Could you check a few things on this model? Use its own coordinates, in mm. A direction names the side the tool comes from. Give positions to 0.01 mm unless a question says otherwise; leave off trailing zeros. Order: outer loops, then holes, each group sorted by start corner. A loop starts at its lowest first (then second) coordinate and runs counter-clockwise, first axis right, second up.
from build123d import *

# Parameters (mm, degrees)
ESQUISSE1_R             = 1.55
BOSS_EXTRU_1_DEPTH      = 8
ENL_V_MAT_EXTRU_1_DEPTH = 4
ESQUISSE3_R             = 4
ENL_V_MAT_EXTRU_2_DEPTH = 38


with BuildPart() as part:
    # Esquisse1 → Boss.-Extru.1 (new body)
    with BuildSketch(Plane.XY):
        with BuildLine():
            Line((-2.034299831, 64.480985332), (56.965700169, 64.480985332))
            Line((56.965700169, 64.480985332), (56.965700169, 46.626034607))
            ThreePointArc((56.965700169, 46.626034607), (56.941837013, 44.504848488), (59.063023131, 44.480985332))
            Line((59.063023131, 44.480985332), (62.935403121, 44.480985332))
            ThreePointArc((62.935403121, 44.480985332), (65.056723464, 44.480985332), (65.056723464, 46.602305676))
            Line((65.056723464, 46.602305676), (65.056723464, 64.480985332))
            Line((65.056723464, 64.480985332), (249.965700169, 64.480985332))
            Line((249.965700169, 64.480985332), (249.965700169, 34.480985332))
            Line((249.965700169, 34.480985332), (244.087020512, 34.480985332))
            ThreePointArc((244.087020512, 34.480985332), (241.965700169, 34.480985332), (241.965700169, 32.359664989))
            Line((241.965700169, 32.359664989), (241.965700169, -3.397694324))
            ThreePointArc((241.965700169, -3.397694324), (241.965700169, -5.519014668), (244.087020512, -5.519014668))
            Line((244.087020512, -5.519014668), (249.965700169, -5.519014668))
            Line((249.965700169, -5.519014668), (249.965700169, -35.519014668))
            Line((249.965700169, -35.519014668), (47.965700169, -35.519014668))
            Line((47.965700169, -35.519014668), (47.965700169, 12.359664989))
            ThreePointArc((47.965700169, 12.359664989), (47.965700169, 14.480985332), (45.844379825, 14.480985332))
            Line((45.844379825, 14.480985332), (42.087020512, 14.480985332))
            ThreePointArc((42.087020512, 14.480985332), (39.965700169, 14.480985332), (39.965700169, 12.359664989))
            Line((39.965700169, 12.359664989), (39.965700169, -35.519014668))
            Line((39.965700169, -35.519014668), (-50.034299831, -35.519014668))
            Line((-50.034299831, -35.519014668), (-50.034299831, 22.512874652))
            Line((-50.034299831, 22.512874652), (-2.034299831, 64.480985332))
        make_face()
        with Locations((245.965700169, 49.480985332)):
            Circle(ESQUISSE1_R, mode=Mode.SUBTRACT)
        with Locations((245.965700169, -20.519014668)):
            Circle(ESQUISSE1_R, mode=Mode.SUBTRACT)
        with Locations((43.965700169, 39.480985332)):
            Circle(ESQUISSE1_R, mode=Mode.SUBTRACT)
    extrude(amount=BOSS_EXTRU_1_DEPTH)

    # Esquisse2 → Enlèv. mat.-Extru.1 (cut)
    with BuildSketch(Plane(origin=(0, 0, 0), x_dir=(-1, 0, 0), z_dir=(0, 0, -1))):
        with BuildLine():
            Line((-245.965700169, 64.480985332), (-60.965700169, 64.480985332))
            Line((-60.965700169, 64.480985332), (-60.965700169, 52.480985332))
            Line((-60.965700169, 52.480985332), (-243.844379825, 52.480985332))
            ThreePointArc((-243.844379825, 52.480985332), (-245.965700169, 52.480985332), (-245.965700169, 54.602305676))
            Line((-245.965700169, 54.602305676), (-245.965700169, 64.480985332))
        make_face()
    extrude(amount=-ENL_V_MAT_EXTRU_1_DEPTH, mode=Mode.SUBTRACT)

    # Esquisse3 → Enlèv. mat.-Extru.2 (cut)
    with BuildSketch(Plane(origin=(0, 0, 0), x_dir=(-1, 0, 0), z_dir=(0, 0, -1))):
        with Locations((30.034299831, -15.519014668)):
            Circle(ESQUISSE3_R)
    extrude(amount=-ENL_V_MAT_EXTRU_2_DEPTH, mode=Mode.SUBTRACT)


solid = part.part
Item 1: Imagine slicing it at A-A on z = 2.75. Give the number of separate pieces and of enclosed holes in the cut face, then the cut area to 3 significant figures.
Findings:
separate pieces: 1
enclosed holes: 4
area: 25,900 mm2
Item 2: For pin 1 (1.1 mm diameter, centred on x = 44, z = 4, fed in from -Y); pin 2 (1.2 mm diameter, centred on y = 60.5, z = 2.5, fed in from -X); pin 3 (3 mm diameter, centred on x = 133, z = 2, fed in from +Y), each with a flat end and sliding along its axis, tell me the tip position at first contact or that it passes through.
Findings:
pin 1: stops at y = 14.48
pin 2: stops at x = -7.27
pin 3: stops at y = 52.48
Item 3: Please list where these lines run through material, in increasing order: line 1 along X through (y, z) = (-20.5, 7.25); line 2 along X through (y, z) = (3.5, 5.25); line 3 along Y through (x, z) = (185.5, 1.75).
Findings:
line 1: x = -50.03 to 39.97, 47.97 to 244.42, 247.52 to 249.97
line 2: x = -50.03 to 39.97, 47.97 to 241.97
line 3: y = -35.52 to 52.48
Item 4: Imagine slicing it at B-B on x = 210.5. List the corners of the cut face in (y, z) for me.
Findings:
outline: (-35.52, 0) - (52.48, 0) - (52.48, 4) - (64.48, 4) - (64.48, 8) - (-35.52, 8) - close
Item 5: We'd pull the mould along Y, two halves only. Please class faces 1 (the flat face through (241.966, 15, 4)), 2 (the flat face through (249.966, 50, 4)), 3 (the flat face through (150, -35.519, 4)): +Y half, -Y half, draft (parallel to the pull), parting line (faces both ways), or undercut.
Findings:
face 1: undercut
face 2: draft
face 3: -Y half
Item 6: For faces 4 (the flat face through (102, 15, 0)), 5 (the flat face through (249.966, -20, 4)), 6 (the flat face through (47.966, -12, 4)), 7 (the flat face through (65.057, 53, 5)), 8 (the flat face through (247, -5.519, 4)), which set-ups out of +Z, -Z, +X, -X, +Y, -Y let a thin tool reach every point of the face, with its end or its side?
Findings:
face 4: -Z, +X, -X, +Y, -Y
face 5: +Z, -Z, +X, +Y, -Y
face 6: +Z, -Z, -Y
face 7: +Z, -Z, +Y
face 8: +Z, -Z, +X
